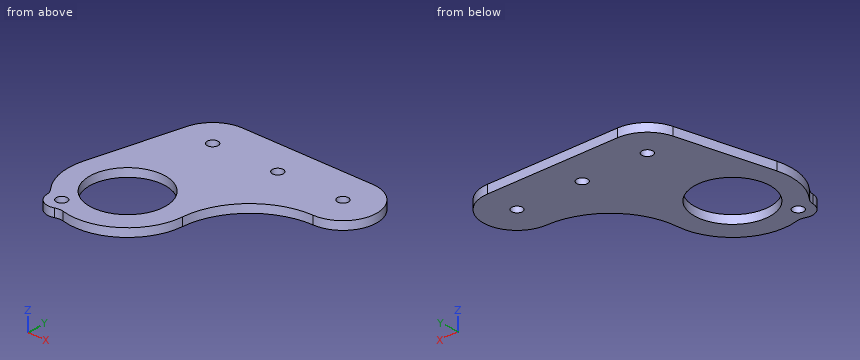
Autodesk Inventor part; units mm, degrees
ref_plane "YZ Plane" through (0, 0, 0) normal (1, 0, 0) x (0, 1, 0)
ref_plane "XZ Plane" through (0, 0, 0) normal (0, 1, 0) x (-1, 0, 0)
ref_plane "XY Plane" through (0, 0, 0) normal (0, 0, 1) x (1, 0, 0)
sketch "Sketch1" plane through (0, 0, 0) normal (0, 0, 1) x (1, 0, 0)
  circle A0 centre (0, 0) radius 14.2875
  circle A1 centre (-1.4096, 37.9321) radius 2.0701
  circle A2 centre (23.9904, 37.9321) radius 2.0701
  circle A3 centre (49.3904, 37.9321) radius 2.0701
  line L0 (-1.4096, 37.9321) -> (49.3904, 37.9321) construction
  circle A4 centre (0, 0) radius 22.225
  line L1 (-1.4096, 37.9321) -> (49.3904, 37.9321) construction
  line L2 (-1.4096, 25.2321) -> (49.3904, 25.2321) construction
  line L3 (49.3904, 50.6321) -> (-1.4096, 50.6321)
  arc A5 (-1.4096, 50.6321) -> (-1.4096, 25.2321) centre (-1.4096, 37.9321) ccw
  arc A6 (49.3904, 25.2321) -> (49.3904, 50.6321) centre (49.3904, 37.9321) ccw
  line L4 (-21.7062, 4.7742) -> (-13.8131, 40.6603)
  arc A7 (49.3904, 25.2321) -> (22.2073, -0.887) centre (49.3904, -1.9727) ccw
  line L5 (-10.67, -20.3) -> (-13.7684, -18.3404) construction
  line L6 (-13.7684, -18.3404) -> (-13.6206, -14.6772) construction
  line L7 (-13.6206, -14.6772) -> (-10.3742, -12.9737) construction
  line L8 (-10.3742, -12.9737) -> (-7.2757, -14.9333) construction
  line L9 (-7.2757, -14.9333) -> (-7.4236, -18.5965) construction
  line L10 (-7.4236, -18.5965) -> (-10.67, -20.3) construction
  circle A8 centre (0, 0) radius 16.51 construction
  circle A9 centre (-10.5221, -16.6369) radius 2.0701
  line L11 (-10.5221, -16.6369) -> (0, 0) construction
  circle A10 centre (-10.5221, -16.6369) radius 5.3975
  arc A11 (-15.8971, -17.1289) -> (-17.1155, -14.1778) centre (-21.2721, -17.621) ccw
  arc A12 (-5.4746, -21.5402) -> (-8.6631, -21.7041) centre (-6.8041, -26.7714) ccw
  circle A13 centre (-10.5221, -16.6369) radius 4.0005 construction
  point P0 (23.9904, 37.9321)
  point P1 (-12.2192, -19.3202)
  dimension "d0" = 25.4
  dimension "d2" = 62.2757
  dimension "d3" = 37.9583
  dimension "d4" = 4.1402
  dimension "d5" = 28.575
  dimension "d6" = 44.45
  dimension "d7" = 25.4
  dimension "d10" = 6.35
  dimension "d11" = 33.02
  dimension "d12" = 8.001
extrude "Extrusion1" add sketch "Sketch1" along normal blind 3.175
sketch "Sketch2" plane through (0, 0, 3.175) normal (0, 0, 1) x (1, 0, 0)
  arc A0 (-15.8971, -17.1289) -> (-8.6631, -21.7041) centre (-10.5221, -16.6369) ccw
  arc A1 (-5.4746, -21.5402) -> (-8.6631, -21.7041) centre (-6.8041, -26.7714) ccw
  arc A2 (-5.4746, -21.5402) -> (22.2073, -0.887) centre (0, 0) ccw
  arc A3 (49.3904, 25.2321) -> (22.2073, -0.887) centre (49.3904, -1.9727) ccw
  arc A4 (49.3904, 25.2321) -> (49.3904, 50.6321) centre (49.3904, 37.9321) ccw
  line L0 (49.3904, 50.6321) -> (-1.4096, 50.6321)
  arc A5 (-1.4096, 50.6321) -> (-13.8131, 40.6603) centre (-1.4096, 37.9321) ccw
  line L1 (-13.8131, 40.6603) -> (-21.7062, 4.7742)
  arc A6 (-21.7062, 4.7742) -> (-17.1155, -14.1778) centre (0, 0) ccw
  arc A7 (-15.8971, -17.1289) -> (-17.1155, -14.1778) centre (-21.2721, -17.621) ccw
  circle A8 centre (0, 0) radius 14.2875
  circle A9 centre (-1.4096, 37.9321) radius 2.0701
  circle A10 centre (49.3904, 37.9321) radius 2.0701
  circle A11 centre (23.9904, 37.9321) radius 2.0701
  circle A12 centre (-10.5221, -16.6369) radius 2.0701
properties part number "Intake Joint Holder Using 1__16 Gray Tinted Polycarbonate Sheet (36 x 72) (217-6627)" material "Polycarbonate, Clear"
CAD build for the part. Positions are in the model's coordinates, mm. Coordinates: 2 decimals unless noted, no trailing zeros. Write each loop counter-clockwise with the first axis right and the second up, starting at its lowest first coordinate (ties: lowest second). Pieces come first, ordered by that corner, then holes. Notation, with made-up numbers: (38.5, 72) - (68.5, 72) arc R12 cw to (68.5, 93) - close; hole circle Ø6 at (-23.5, 87.5). An arc over 180 degrees is marked (long way). Use a Markdown table: item, result. Add a question column.
Item 1: Band-saw the part on B-B, the plane x = 2.5. Give the cut face in (y, z) (3 decimals).
Item 2: Band-saw the part on D-D, the plane x = -10. Give the cut face in (y, z) (3 decimals).
Item 3: Band-saw the part on A-A, the plane y = 8.5. Give the cut face in (x, z) (3 decimals).
Item 4: Band-saw the part on C-C, the plane z = 2. Give the number of separate pieces and of enclosed holes in the cut face, and give its area (3 significant figures).
Item 5: Drill centre lines: L1, parallel to Y at x = 0, z = 1.65 (1 decimal); L2, parallel to X at y = -0.5, z = 0.5; L3, parallel to X at y = 0, z = 0.8 (1 decimal). Where is each one in solid material? Low to high. Write a range as from..to.
Item 6: Flat gauge pins, fed straight in: pin 1 (3.5 mm diameter, centred on x = 49.39, y = 37.93, fed in from +Z); pin 2 (8 mm diameter, centred on x = 2.5, y = 25.5, fed in from -Z). Where does each tip first touch, or does it go through?
Numbers:
| question | item | result |
|---|---|---|
| 1 | outline | (-22.084, 0) - (-14.067, 0) - (-14.067, 3.175) - (-22.084, 3.175) - close; (14.067, 0) - (50.632, 0) - (50.632, 3.175) - (14.067, 3.175) - close |
| 2 | outline | (-22.009, 0) - (-18.64, 0) - (-18.64, 3.175) - (-22.009, 3.175) - close; (-14.634, 0) - (-10.205, 0) - (-10.205, 3.175) - (-14.634, 3.175) - close; (10.205, 0) - (47.286, 0) - (47.286, 3.175) - (10.205, 3.175) - close |
| 3 | outline | (-20.887, 0) - (-11.484, 0) - (-11.484, 3.175) - (-20.887, 3.175) - close; (11.484, 0) - (24.282, 0) - (24.282, 3.175) - (11.484, 3.175) - close |
| 4 | separate pieces | 1 |
| 4 | enclosed holes | 5 |
| 4 | area | 3,180 mm2 |
| 5 | L1 | -22.2..-14.3, 14.3..36.4, 39.4..50.6 |
| 5 | L2 | -22.22..-14.28, 14.28..22.23 |
| 5 | L3 | -22.2..-14.3, 14.3..22.3 |
| 6 | pin 1 | through |
| 6 | pin 2 | z = 0 |
